The drawing under review shows one solid part. Ordinate dimensions are in mm from its lowest x, y, z. Coordinates: 2 decimals unless noted, no trailing zeros. Loops run counter-clockwise (first coordinate to the right, second up) from the corner with the lowest first, then second, coordinate; pieces in that order, holes last. Notation, with made-up numbers: (19.25, 46) -> (50.25, 46) arc R27 ccw to (50.25, 68) -> close; hole circle Ø5 at (12, 21). An arc over 180 degrees is marked (long way). Use a Markdown table: item, result.
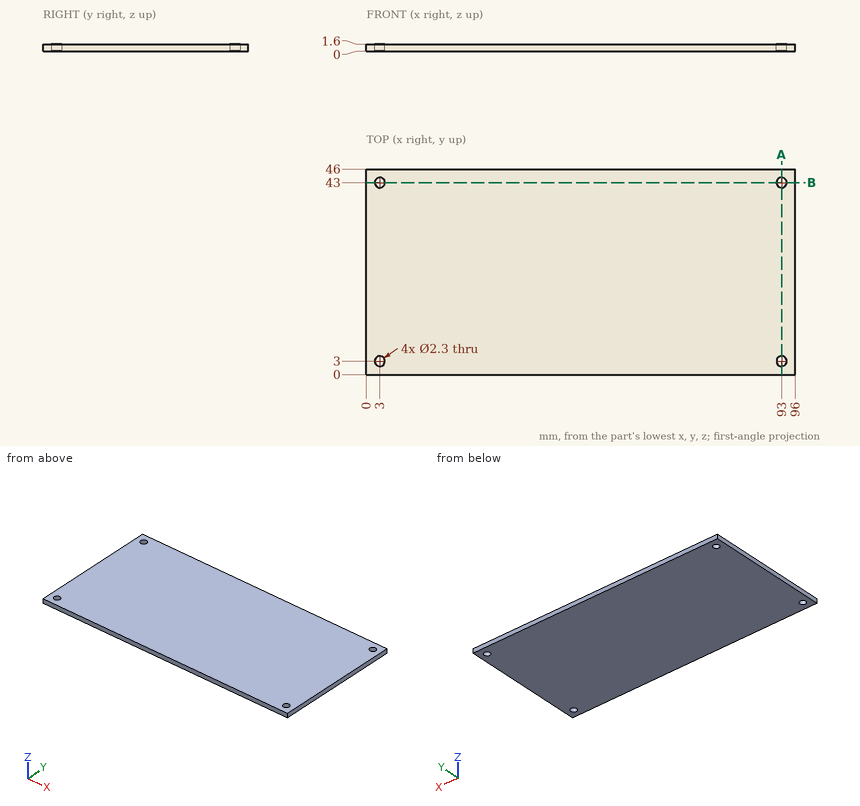
(1) For line 1 along X through (y, z) = (43, 0.7); line 2 along Y through (x, z) = (3, 1.15), list the stretches that pass through material, from the lowest coordinate up.
Found:
| item | result |
|---|---|
| line 1 | x = 0 to 1.85, 4.15 to 91.85, 94.15 to 96 |
| line 2 | y = 0 to 1.85, 4.15 to 41.85, 44.15 to 46 |
(2) Take a section at A-A on x = 93. Write out the cut boundary in (y, z).
Found:
| item | result |
|---|---|
| outline | (0, 0) -> (1.85, 0) -> (1.85, 1.6) -> (0, 1.6) -> close; (4.15, 0) -> (41.85, 0) -> (41.85, 1.6) -> (4.15, 1.6) -> close; (44.15, 0) -> (46, 0) -> (46, 1.6) -> (44.15, 1.6) -> close |
(3) Take a section at B-B on y = 43. Write out the cut boundary in (x, z), plus the area to 3 significant figures.
Found:
| item | result |
|---|---|
| outline | (0, 0) -> (1.85, 0) -> (1.85, 1.6) -> (0, 1.6) -> close; (4.15, 0) -> (91.85, 0) -> (91.85, 1.6) -> (4.15, 1.6) -> close; (94.15, 0) -> (96, 0) -> (96, 1.6) -> (94.15, 1.6) -> close |
| area | 146 mm^2 |
